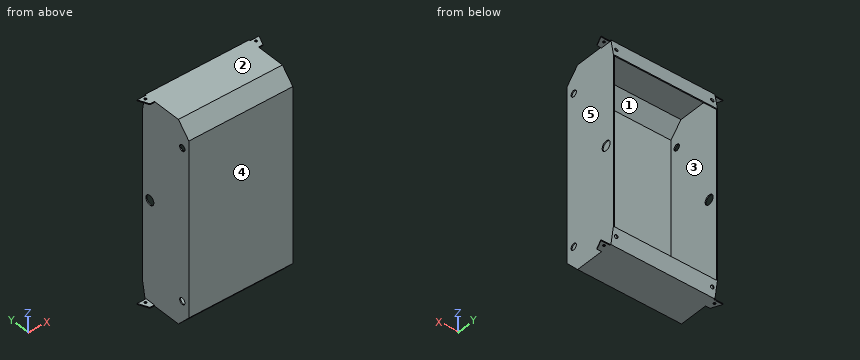
```python
from build123d import *

# Parameters (mm, degrees)
ESQUISSE1_W             = 208.5
ESQUISSE1_H             = 111
BOSS_EXTRU_1_DEPTH      = 404
ESQUISSE3_W             = 18
ESQUISSE3_H             = 400
ENL_V_MAT_EXTRU_2_DEPTH = 475.36747359
ENL_V_MAT_EXTRU_3_DEPTH = 477.276442835
COQUE2_START            = 2
COQUE2_DEPTH            = 204.5
ENL_V_MAT_EXTRU_4_REACH = 478.276
ESQUISSE5_W             = 204.5
ESQUISSE5_H             = 339.253793908
D_GAGEMENT_1_41_D       = 6.7564
D_GAGEMENT_1_41_DEPTH   = 2
D_GAGEMENT_1_42_D       = 6.7564
D_GAGEMENT_1_42_DEPTH   = 2
ESQUISSE10_R            = 9.525
ESQUISSE10_R_2          = 6.35
ENL_V_MAT_EXTRU_5_DEPTH = 477.276442835
ENL_V_MAT_EXTRU_6_REACH = 478.276
ESQUISSE11_R            = 2.38125
ENL_V_MAT_EXTRU_7_REACH = 478.276
ESQUISSE12_R            = 2.38125


# Read off the part's stored shape, not the designer's step: Coque2
with BuildPart() as part:
    # Esquisse1 → Boss.-Extru.1 (new body)
    with BuildSketch(Plane.XY):
        with Locations((104.25, 55.5)):
            Rectangle(ESQUISSE1_W, ESQUISSE1_H)
        Polygon((0, 102.5), (-18, 102.5), (-9, 82.5), (0, 82.5), align=None)
        Polygon((208.5, 102.5), (226.5, 102.5), (217.5, 82.5), (208.5, 82.5), align=None)
    extrude(amount=-BOSS_EXTRU_1_DEPTH)

    # Esquisse3 → Enlèv. mat.-Extru.2 (cut, through all)
    with BuildSketch(Plane(origin=(0, 102.5, 0), x_dir=(1, 0, 0), z_dir=(0, 1, 0))):
        with Locations((-9, 202)):
            Rectangle(ESQUISSE3_W, ESQUISSE3_H)
        with Locations((217.5, 202)):
            Rectangle(ESQUISSE3_W, ESQUISSE3_H)
    extrude(amount=-ENL_V_MAT_EXTRU_2_DEPTH, mode=Mode.SUBTRACT)

    # Esquisse4 → Enlèv. mat.-Extru.3 (cut, through all)
    with BuildSketch(Plane.ZY):
        Polygon((0, 105), (-32.373103046, 111), (0, 111), align=None)
        Polygon((-404, 105), (-371.626896954, 111), (-404, 111), align=None)
        Polygon((0, 25), (-27.276363394, 0), (0, 0), align=None)
        Polygon((-404, 25), (-376.723636606, 0), (-404, 0), align=None)
    extrude(amount=-ENL_V_MAT_EXTRU_3_DEPTH, mode=Mode.SUBTRACT)

    # Coque2 outline → Coque2 (cut)
    with BuildSketch(Plane.YZ.offset(COQUE2_START)):
        Polygon((25.87988269, -402), (103.336617558, -402), (109, -371.443122771), (109, -32.556877229), (103.336617558, -2), (25.87988269, -2), (2, -28.054254322), (2, -375.945745678), align=None)
    extrude(amount=COQUE2_DEPTH, mode=Mode.SUBTRACT)

    # Esquisse5 → Enlèv. mat.-Extru.4 (cut, up to next)
    with BuildSketch(Plane(origin=(0, 111, 0), x_dir=(1, 0, 0), z_dir=(0, 1, 0)), mode=Mode.PRIVATE) as enl_v_mat_extru_4_sk1:
        with Locations((104.25, 202)):
            Rectangle(ESQUISSE5_W, ESQUISSE5_H)
    enl_v_mat_extru_4_tool1 = extrude(enl_v_mat_extru_4_sk1.sketch, amount=-ENL_V_MAT_EXTRU_4_REACH, mode=Mode.PRIVATE) & part.part
    add(enl_v_mat_extru_4_tool1.solids().sort_by_distance((104.25, 111, -202))[0], mode=Mode.SUBTRACT)

    # Dégagement 1/41
    with Locations(Plane(origin=(0, 101.512972391, 18.814317351), x_dir=(1, 0, 0), z_dir=(0, 0.983254907563956, 0.18223552549214056))):
        with Locations((8, 37.059155773), (200.5, 37.059155773)):
            Hole(D_GAGEMENT_1_41_D / 2, depth=D_GAGEMENT_1_41_DEPTH)

    # Dégagement 1/42
    with Locations(Plane(origin=(0, 173.903298199, -32.231071199), x_dir=(1, 0, 0), z_dir=(0, 0.983254907563956, -0.18223552549214078))):
        with Locations((8, 360.175826883), (200.5, 360.175826883)):
            Hole(D_GAGEMENT_1_42_D / 2, depth=D_GAGEMENT_1_42_DEPTH)

    # Esquisse10 → Enlèv. mat.-Extru.5 (cut, through all)
    with BuildSketch(Plane.ZY):
        with Locations((-202, 93.525)):
            Circle(ESQUISSE10_R)
        with Locations((-353.2, 15.75)):
            Circle(ESQUISSE10_R_2)
        with Locations((-50.8, 15.75)):
            Circle(ESQUISSE10_R_2)
    extrude(amount=-ENL_V_MAT_EXTRU_5_DEPTH, mode=Mode.SUBTRACT)

    # Esquisse11 → Enlèv. mat.-Extru.6 (cut, up to next)
    with BuildSketch(Plane.XY, mode=Mode.PRIVATE) as enl_v_mat_extru_6_sk1:
        with Locations((-6.74, 96.27)):
            Circle(ESQUISSE11_R)
    enl_v_mat_extru_6_tool1 = extrude(enl_v_mat_extru_6_sk1.sketch, amount=-ENL_V_MAT_EXTRU_6_REACH, mode=Mode.PRIVATE) & part.part
    # Esquisse11 → Enlèv. mat.-Extru.6 (cut, up to next)
    with BuildSketch(Plane.XY, mode=Mode.PRIVATE) as enl_v_mat_extru_6_sk2:
        with Locations((215.24, 96.27)):
            Circle(ESQUISSE11_R)
    enl_v_mat_extru_6_tool2 = extrude(enl_v_mat_extru_6_sk2.sketch, amount=-ENL_V_MAT_EXTRU_6_REACH, mode=Mode.PRIVATE) & part.part
    add(enl_v_mat_extru_6_tool1.solids().sort_by_distance((-6.74, 96.27, 0))[0], mode=Mode.SUBTRACT)
    add(enl_v_mat_extru_6_tool2.solids().sort_by_distance((215.24, 96.27, 0))[0], mode=Mode.SUBTRACT)

    # Esquisse12 → Enlèv. mat.-Extru.7 (cut, up to next)
    with BuildSketch(Plane(origin=(0, 0, -404), x_dir=(-1, 0, 0), z_dir=(0, 0, -1)), mode=Mode.PRIVATE) as enl_v_mat_extru_7_sk1:
        with Locations(Location((-215.24, 96.27, 0), (0, 0, 180))):
            Circle(ESQUISSE12_R)
    enl_v_mat_extru_7_tool1 = extrude(enl_v_mat_extru_7_sk1.sketch, amount=-ENL_V_MAT_EXTRU_7_REACH, mode=Mode.PRIVATE) & part.part
    # Esquisse12 → Enlèv. mat.-Extru.7 (cut, up to next)
    with BuildSketch(Plane(origin=(0, 0, -404), x_dir=(-1, 0, 0), z_dir=(0, 0, -1)), mode=Mode.PRIVATE) as enl_v_mat_extru_7_sk2:
        with Locations(Location((6.74, 96.27, 0), (0, 0, 180))):
            Circle(ESQUISSE12_R)
    enl_v_mat_extru_7_tool2 = extrude(enl_v_mat_extru_7_sk2.sketch, amount=-ENL_V_MAT_EXTRU_7_REACH, mode=Mode.PRIVATE) & part.part
    add(enl_v_mat_extru_7_tool1.solids().sort_by_distance((215.24, 96.27, -404))[0], mode=Mode.SUBTRACT)
    add(enl_v_mat_extru_7_tool2.solids().sort_by_distance((-6.74, 96.27, -404))[0], mode=Mode.SUBTRACT)


solid = part.part
```
Verification items for the finished model (mm, model axes). Face numbers are marked on the shaded views. A direction names the side the tool comes from. Round coordinates to 2 decimals unless told otherwise and drop trailing zeros. Write each loop counter-clockwise with the first axis right and the second up, starting at its lowest first coordinate (ties: lowest second). Pieces come first, ordered by that corner, then holes.
1. Section check C-C on x = 21. Enter the section's corners in (y, z), plus the area to 3 significant figures.
2. Section check D-D on z = -353.2. Enter the section's corners in (x, y), plus the area to 3 significant figures.
3. Section check A-A on z = -202. Enter the section's corners in (x, y), plus the area to 3 significant figures.
4. Draft check along Y on the marked faces 3, 4 and 5. Enter one of: +Y half, -Y half, draft (parallel to the pull), parting line (faces both ways), or undercut.
5. Section check B-B on y = 73. Enter the section's corners in (x, z).
6. Access from +Z, -Z, +X, -X, +Y, -Y to the whole of each face (thin tool, end or side, straight path). Record for the marked faces 1 and 2.
7. Scan lines: L1, parallel to X at y = 94, z = -173; L2, parallel to Z at x = 104.5, y = 71.5; L3, parallel to X at y = 96.27, z = -403.45. Record each from-to range of solid material in increasing order.
8. Gauge pin test, flat ends, axial feed: P1, Ø5, axis at x = 161.5, z = -321, coming from the +Y side; P2, Ø16.5, axis at y = 15.75, z = -50.8, coming from the -X side. Record the tip position at first contact, or that the pin passes through.
Answer:
1. outline: (0, -376.72) - (25, -404) - (105, -404) - (111, -371.63) - (108.97, -371.63) - (103.34, -402) - (25.88, -402) - (2, -375.95) - (2, -28.05) - (25.88, -2) - (103.34, -2) - (108.97, -32.37) - (111, -32.37) - (105, 0) - (25, 0) - (0, -27.28) - close
1. area: 1,280 mm2
2. outline: (0, 0) - (208.5, 0) - (208.5, 9.4) - (206.5, 9.4) - (206.5, 2) - (2, 2) - (2, 9.4) - (0, 9.4) - close; (0, 22.1) - (2, 22.1) - (2, 111) - (0, 111) - close; (206.5, 22.1) - (208.5, 22.1) - (208.5, 111) - (206.5, 111) - close
2. area: 802 mm2
3. outline: (0, 0) - (208.5, 0) - (208.5, 84) - (206.5, 84) - (206.5, 2) - (2, 2) - (2, 84) - (0, 84) - close; (0, 103.05) - (2, 103.05) - (2, 111) - (0, 111) - close; (206.5, 103.05) - (208.5, 103.05) - (208.5, 111) - (206.5, 111) - close
3. area: 777 mm2
4. face 3: undercut
4. face 4: -Y half
4. face 5: draft
5. outline: (0, -404) - (208.5, -404) - (208.5, 0) - (0, 0) - close; hole (2, -402) - (206.5, -402) - (206.5, -2) - (2, -2) - close
6. face 1: none
6. face 2: +Z, +X, -X, +Y, -Y
7. L1: x = 0 to 2, 206.5 to 208.5
7. L2: z = -404 to -402, -2 to 0
7. L3: x = -15.2 to -9.12, -4.36 to 212.86, 217.62 to 223.7
8. P1: stops at y = 2
8. P2: stops at x = 0
